```python
from build123d import *

# Parameters (mm, degrees)
F1_DEPTH       = 25
F5_D           = 5.5
F5_START       = 0.4196012
F5_CBORE_D     = 10
F5_CBORE_DEPTH = 2.5
F7_D           = 5.5
F7_CBORE_D     = 10
F7_CBORE_DEPTH = 2.5
F8_R           = 5
F9_R           = 10
F10_R          = 10


with BuildPart() as f1:
    # F0 (on Front) → F1 (new body, symmetric)
    with BuildSketch(Plane.XZ):
        with BuildLine():
            Line((-55, -20), (-55, -25))
            Line((-55, -25), (-25, -25))
            Line((-25, -25), (-25, 0))
            ThreePointArc((-25, 0), (0, 25), (25, 0))
            Line((25, 0), (25, -25))
            Line((25, -25), (55, -25))
            Line((55, -25), (55, -20))
            Line((55, -20), (30, -20))
            Line((30, -20), (30, 0))
            ThreePointArc((30, 0), (0, 30), (-30, 0))
            Line((-30, 0), (-30, -20))
            Line((-30, -20), (-55, -20))
        make_face()
    extrude(amount=F1_DEPTH, both=True)

    # F5 (through all)
    # its depths count from where the whole tool has entered the part; down to there all is cleared
    with Locations(Plane.XY.offset(30).offset(-F5_START)):
        with Locations((0, 0)):
            CounterBoreHole(F5_D / 2, F5_CBORE_D / 2, F5_CBORE_DEPTH)

    # F7 (through all)
    with Locations(Plane.XY.offset(-20)):
        with Locations((-42.5, 0), (42.5, 0)):
            CounterBoreHole(F7_D / 2, F7_CBORE_D / 2, F7_CBORE_DEPTH)

    # F8
    f8_edges = [f1.edges().sort_by_distance(p)[0] for p in [
        (30, 0, -20),
        (-30, 0, -20),
    ]]
    fillet(f8_edges, radius=F8_R)

    # F9
    f9_edges = [f1.edges().sort_by_distance(p)[0] for p in [
        (25, 0, -25),
        (-25, 0, -25),
    ]]
    fillet(f9_edges, radius=F9_R)

    # F10
    f10_edges = [f1.edges().sort_by_distance(p)[0] for p in [
        (-55, -25, -22.5),
        (55, -25, -22.5),
        (55, 25, -22.5),
        (-55, 25, -22.5),
    ]]
    fillet(f10_edges, radius=F10_R)


solid = f1.part
```
The model under review builds one solid part; all positions refer to its coordinate system, in mm. A direction names the side the tool comes from. Coordinates: 2 decimals unless noted, no trailing zeros. Order: outer loops, then holes, each group sorted by start corner. A loop starts at its lowest first (then second) coordinate and runs counter-clockwise, first axis right, second up. Notation, with made-up numbers: (-13.5, 50) -> (37.5, 50) arc R29 cw to (37.5, 86) -> close; hole circle Ø4 at (46, 32.5). An arc over 180 degrees is marked (long way). Answer in a Markdown table with one row per item. Add a question column.
Item 1: We need section A-A on x = 42.5. Write out the cut boundary in (y, z), plus the area to 3 significant figures.
Item 2: We need section D-D on x = 0. Write out the cut boundary in (y, z), plus the area to 3 significant figures.
Item 3: Machinability: for faces 1 (the cylindrical face through (-27.85, -0.35, -21.99)), 2 (the cylindrical face through (-51.99, 22.15, -22.54)), 3 (the flat face through (-55, 0, -22)), 4 (the flat face through (-30, 0, -7)), 5 (the cylindrical face through (37.505, 0.22, -21.232)), which of the approach directions +Z, -Z, +X, -X, +Y, -Y give a long, thin tool a straight path to every point of the face, cutting with its end or side? Answer none if there is none.
Item 4: We need section C-C on z = -10. Write out the cut boundary in (x, y), plus the area to 3 significant figures.
Item 5: We need section B-B on y = 7. Write out the cut boundary in (x, z), plus the area to 3 significant figures.
Item 6: To check wall thickness, follow probe 1 along Y at (x, z) = (-42, -21); probe 2 along Y at (x, z) = (-42.5, -23.7); probe 3 along X at (y, z) = (-8, -1). State the ranges of each line that lie inside material, in increasing order.
Item 7: Mouldability with a two-part tool opening along X and no side actions: class faces 6 (the flat face through (30, 0, -8)), 7 (the cylindrical face through (-52.15, -21.99, -22.54)), 8 (the cylindrical face through (-47.495, 0.22, -21.232)) as +X half, -X half, draft (parallel to the pull), parting line (faces both ways), or undercut.
Item 8: Clearance check with flat-ended pins moving along their axes: pin 1 (3 mm diameter, centred on y = -19, z = 5.5, fed in from -X); pin 2 (3.5 mm diameter, centred on x = -42.5, y = 0, fed in from -Z); pin 3 (1.5 mm diameter, centred on x = -32.5, y = -8, fed in from +Z); pin 4 (3 mm diameter, centred on y = -15.5, z = -1.5, fed in from -X). State where each tip first meets the part, or that it passes through.
Final values:
| question | item | result |
|---|---|---|
| 1 | outline | (-25, -25) -> (-2.75, -25) -> (-2.75, -22.5) -> (-5, -22.5) -> (-5, -20) -> (-25, -20) -> close; (2.75, -25) -> (25, -25) -> (25, -20) -> (5, -20) -> (5, -22.5) -> (2.75, -22.5) -> close |
| 1 | area | 211 mm2 |
| 2 | outline | (-25, 25) -> (-2.75, 25) -> (-2.75, 27.08) -> (-5, 27.08) -> (-5, 30) -> (-25, 30) -> close; (2.75, 25) -> (25, 25) -> (25, 30) -> (5, 30) -> (5, 27.08) -> (2.75, 27.08) -> close |
| 2 | area | 209 mm2 |
| 3 | face 1 | -Z, +Y, -Y |
| 3 | face 2 | +Z, -Z, -X, +Y |
| 3 | face 3 | +Z, -Z, -X, +Y, -Y |
| 3 | face 4 | +Z, -X, +Y, -Y |
| 3 | face 5 | +Z |
| 4 | outline | (-30, -25) -> (-25, -25) -> (-25, 25) -> (-30, 25) -> close; (25, -25) -> (30, -25) -> (30, 25) -> (25, 25) -> close |
| 4 | area | 500 mm2 |
| 5 | outline | (-55, -25) -> (-35, -25) arc R10 ccw to (-25, -15) -> (-25, 0) arc R25 cw to (25, 0) -> (25, -15) arc R10 ccw to (35, -25) -> (55, -25) -> (55, -20) -> (35, -20) arc R5 cw to (30, -15) -> (30, 0) arc R30 ccw to (-30, 0) -> (-30, -15) arc R5 cw to (-35, -20) -> (-55, -20) -> close |
| 5 | area | 900 mm2 |
| 6 | probe 1 | y = -25 to -4.97, 4.97 to 25 |
| 6 | probe 2 | y = -25 to -2.75, 2.75 to 25 |
| 6 | probe 3 | x = -30 to -25, 25 to 30 |
| 7 | face 6 | +X half |
| 7 | face 7 | -X half |
| 7 | face 8 | undercut |
| 8 | pin 1 | stops at x = -29.73 |
| 8 | pin 2 | passes through |
| 8 | pin 3 | stops at z = -18.8 |
| 8 | pin 4 | stops at x = -30 |
